Work out the finished part from the listing and answer in its coordinate system (mm). A direction names the side the tool comes from. Round coordinates to 2 decimals unless told otherwise and drop trailing zeros. Write each loop counter-clockwise with the first axis right and the second up, starting at its lowest first coordinate (ties: lowest second). Pieces come first, ordered by that corner, then holes. Notation, with made-up numbers: (45, -14.75) - (69, -14.75) arc R17 cw to (69, -0.75) - close; hole circle Ø4 at (63, 18.5). An arc over 180 degrees is marked (long way). Answer as a JSON object with one key per item and string values.
Autodesk Inventor part; units mm, degrees
ref_plane "YZ Plane" through (0, 0, 0) normal (1, 0, 0) x (0, 1, 0)
ref_plane "XZ Plane" through (0, 0, 0) normal (0, 1, 0) x (-1, 0, 0)
ref_plane "XY Plane" through (0, 0, 0) normal (0, 0, 1) x (1, 0, 0)
sketch "Skizze1" plane through (0, 0, 0) normal (0, 1, 0) x (-1, 0, 0)
  line L0 (-31.5, 40) -> (31.5, 40)
  line L1 (31.5, 40) -> (31.5, -40)
  line L2 (31.5, -40) -> (-31.5, -40)
  line L3 (-31.5, -40) -> (-31.5, 40)
  line L4 (0, -56) -> (0, 56)
  line L5 (-44.1, 0) -> (44.1, 0)
  circle A0 centre (27, -35) radius 1.6
  circle A1 centre (-27, -35) radius 1.6
  circle A2 centre (-27, -1) radius 1.6
  circle A3 centre (27, -1) radius 1.6
  point P0 (0, 0)
  dimension "d0" = 63
  dimension "d1" = 80
  dimension "d2" = 3.2
  dimension "d3" = 3.2
  dimension "d4" = 27
  dimension "d5" = 27
  dimension "d6" = 5
  dimension "d7" = 5
  dimension "d8" = 3.2
  dimension "d9" = 3.2
  dimension "d10" = 27
  dimension "d11" = 27
  dimension "d12" = 34
  dimension "d13" = 34
extrude "Extrusion1" add sketch "Skizze1" along normal blind 2 contours L0 L4 L5 A2 L3 | L0 L1 L5 A3 L4 | L5 A2 L4 L2 L3 | L5 A3 L1 L2 L4
sketch "Skizze3" plane through (0, 2, 0) normal (0, 1, 0) x (1, 0, 0)
  circle A0 centre (-23, 30) radius 3.5
  circle A1 centre (23, 30) radius 3.5
  circle A2 centre (23, -36) radius 3.5
  circle A3 centre (-23, -36) radius 3.5
  line L0 (0, 56) -> (0, -56)
  line L1 (44.1, 0) -> (-44.1, 0)
  line L2 (31.5, 40) -> (-31.5, 40)
  point P0 (0, 0)
  dimension "d22" = 7
  dimension "d23" = 7
  dimension "d24" = 7
  dimension "d25" = 7
  dimension "d26" = 23
  dimension "d27" = 23
  dimension "d28" = 23
  dimension "d29" = 23
  dimension "d31" = 10
  dimension "d32" = 10
  dimension "d33" = 66
  dimension "d34" = 66
sketch "Skizze2" plane through (0, 0, 0) normal (0, -1, 0) x (1, 0, 0)
  circle A0 centre (27, -1) radius 1.6
  circle A1 centre (27, -35) radius 1.6
  circle A2 centre (-27, -35) radius 1.6
  circle A3 centre (-27, -1) radius 1.6
  circle A4 centre (27, -1) radius 3.5
  circle A5 centre (27, -35) radius 3.5
  circle A6 centre (-27, -1) radius 3.5
  circle A7 centre (-27, -35) radius 3.5
  point P0 (0, 0)
  dimension "d16" = 7
  dimension "d17" = 7
  dimension "d18" = 7
  dimension "d19" = 7
extrude "Extrusion2" add sketch "Skizze2" along normal blind 6.5
extrude "Extrusion3" add sketch "Skizze3" against normal blind 6
sketch "Skizze4" plane through (0, 2, 0) normal (0, 1, 0) x (1, 0, 0)
  arc A0 (23.8957, 33.3835) -> (26.1043, 31.6165) centre (23, 30) ccw
  circle A1 centre (23, -36) radius 3.5
  circle A2 centre (-23, -36) radius 3.5
  arc A3 (-26.1043, 31.6165) -> (-23.8957, 33.3835) centre (-23, 30) ccw
  circle A4 centre (23, 30) radius 2.25
  circle A5 centre (23, -36) radius 2.25
  circle A6 centre (-23, 30) radius 2.25
  circle A7 centre (-23, -36) radius 2.25
  point P0 (0, 0)
  dimension "d37" = 4.5
  dimension "d38" = 4.5
  dimension "d39" = 4.5
  dimension "d40" = 4.5
extrude "Extrusion4" cut sketch "Skizze4" against normal up to surface (6 mm away) contours A4 | A5 | A6 | A7
sketch "Skizze5" plane through (0, 2, 0) normal (0, 1, 0) x (1, 0, 0)
  line L0 (23.5, -32) -> (23.5, 25)
  line L1 (-23.5, 25) -> (-23.5, -32)
  line L2 (31.5, 40) -> (-31.5, 40)
  line L3 (-31.5, -40) -> (31.5, -40)
  line L4 (-31.5, 40) -> (-31.5, -40)
  line L5 (31.5, -40) -> (31.5, 40)
  line L6 (18.5, -32) -> (18.5, -37)
  line L7 (18.5, -37) -> (-18.5, -37)
  line L8 (-18.5, -37) -> (-18.5, -32)
  line L9 (18.5, 25) -> (18.5, 35)
  line L10 (18.5, 35) -> (-18.5, 35)
  line L11 (-18.5, 35) -> (-18.5, 25)
  line L12 (-23.5, -32) -> (-18.5, -32)
  line L13 (18.5, -32) -> (23.5, -32)
  line L14 (23.5, 25) -> (18.5, 25)
  line L15 (-18.5, 25) -> (-23.5, 25)
  point P0 (0, 0)
  dimension "d45" = 8
  dimension "d46" = 8
  dimension "d49" = 3
  dimension "d50" = 13
  dimension "d51" = 13
  dimension "d52" = 13
  dimension "d53" = 13
  dimension "d54" = 5
  dimension "d55" = 8
  dimension "d56" = 8
  dimension "d57" = 15
  dimension "d58" = 15
extrude "Extrusion5" cut sketch "Skizze5" against normal up to surface (2 mm away) contours L13 L6 L7 L8 L12 L1 L15 L11 L10 L9 L14 L0
fillet "Rundung1" radius 3.5 4 edges at (18.5, 1, 32) (18.5, 1, -25) (-18.5, 1, -25) (-18.5, 1, 32)
properties part number "Adapter_PowerManagement"
Item 1: A cutting plane is placed at A-A (y = -5.5). Write down the section's boundary in (x, z).
Results found:
{"outline": "circle Ø7 at (-27, -35); circle Ø7 at (-27, -1); circle Ø7 at (27, -35); circle Ø7 at (27, -1); hole circle Ø3.2 at (-27, -35); hole circle Ø3.2 at (-27, -1); hole circle Ø3.2 at (27, -35); hole circle Ø3.2 at (27, -1)"}
Item 2: A cutting plane is placed at B-B (z = 22.5). Write down the section's boundary in (x, y), and give its area (3 significant figures).
Results found:
{"outline": "(-31.5, 0) - (-23.5, 0) - (-23.5, 2) - (-31.5, 2) - close; (23.5, 0) - (31.5, 0) - (31.5, 2) - (23.5, 2) - close", "area": "32.0 mm²"}
Item 3: Consider line 1 along X through (y, z) = (-1.7, -30); line 2 along Z through (x, y) = (-27, -4.75); line 3 along X through (y, z) = (-4.5, -35). Determine where each line is inside the solid, lowest interval first.
Results found:
{"line 1": "-26.5 to -25.25, -20.75 to -19.5, 19.5 to 20.75, 25.25 to 26.5", "line 2": "-38.5 to -36.6, -33.4 to -31.5, -4.5 to -2.6, 0.6 to 2.5", "line 3": "-30.5 to -28.6, -25.4 to -23.5, 23.5 to 25.4, 28.6 to 30.5"}
Item 4: For faces 4 (the flat face through (18.5, 1, -32)), 5 (the flat face through (-26, -6.5, -37)), 6 (the cylindrical face through (22.54, -1.97, 32.53)), determine the directions among +Z, -Z, +X, -X, +Y, -Y from which every point of the face is accessible in a straight line to the end or side of a thin tool.
Results found:
{"face 4": "+Y, -Y", "face 5": "+Z, -Z, +X, -X, -Y", "face 6": "-Y"}
Item 5: A cutting plane is placed at C-C (x = -1.5). Write down the section's boundary in (y, z).
Results found:
{"outline": "(0, -40) - (2, -40) - (2, -35) - (0, -35) - close; (0, 37) - (2, 37) - (2, 40) - (0, 40) - close"}
Item 6: Each of these flat-tipped pins is pushed along its axis until it touches: P1, Ø4, axis at x = -19.5, z = -21.5, coming from the +Y side; P2, Ø3.5, axis at x = 24.5, z = -29, coming from the -Y side. Where does it stop, or does it pass through?
Results found:
{"P1": "through", "P2": "y = -4"}
Item 7: Determine the mould class of faces 1 (the flat face through (-22.3, -4, 38.3)), 2 (the flat face through (0, 1, 40)), 3 (the cylindrical face through (-23.46, -1.97, 32.53)) for opening direction Z: pulls with the +Z half, pulls with the -Z half, needs draft (parallel to the pull), parting line crosses it, or undercut.
Results found:
{"face 1": "needs draft", "face 2": "pulls with the +Z half", "face 3": "undercut"}
